Part print with two shaded views. Sizes in mm from the minimum x, y, z corner. A direction names the side the tool comes from. Round coordinates to 2 decimals unless told otherwise and drop trailing zeros. Order: outer loops, then holes, each group sorted by start corner. A loop starts at its lowest first (then second) coordinate and runs counter-clockwise, first axis right, second up. Notation, with made-up numbers: M 12.25,84 L 21.25,84 A10 cw 21.25,102 Z; hole C 4.25,88 d4. An arc over 180 degrees is marked long. Put each result on its own line as item: value.
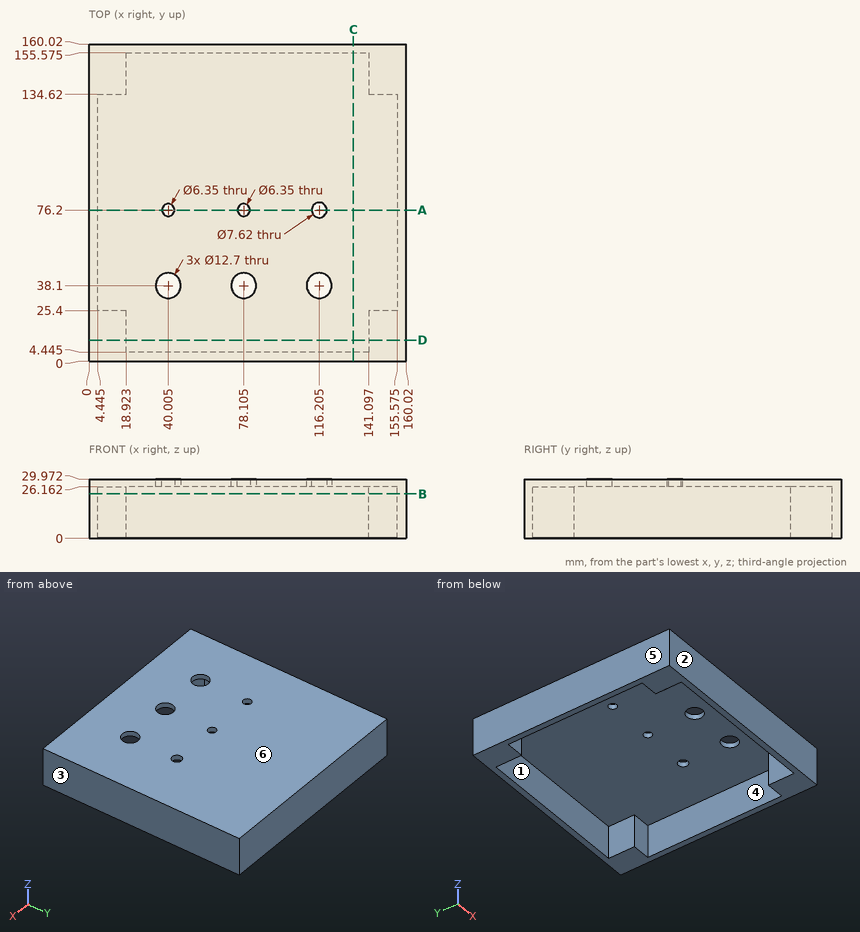
Item 1: Band-saw the part on D-D on y = 10.5. Give the cut face in (x, z), and give its area (3 significant figures).
Answers below:
outline: M 0,0 L 18.92,0 L 18.92,26.16 L 141.1,26.16 L 141.1,0 L 160.02,0 L 160.02,29.97 L 0,29.97 Z
area: 1,600 mm²
Item 2: Band-saw the part on A-A on y = 76.2. Give the cut face in (x, z) (3 decimals).
Answers below:
outline: M 0,0 L 4.445,0 L 4.445,26.162 L 36.83,26.162 L 36.83,29.972 L 0,29.972 Z; M 43.18,26.162 L 74.93,26.162 L 74.93,29.972 L 43.18,29.972 Z; M 81.28,26.162 L 112.395,26.162 L 112.395,29.972 L 81.28,29.972 Z; M 120.015,26.162 L 155.575,26.162 L 155.575,0 L 160.02,0 L 160.02,29.972 L 120.015,29.972 Z
Item 3: Tool access for the marked faces 1 and 2: list every direction of +Z, -Z, +X, -X, +Y, -Y with a clear straight run to the whole face (end or side of a thin tool).
Answers below:
face 1: -Z
face 2: +Z, -Z, +X, -X, -Y
Item 4: Probe line 1 along Y through (x, z) = (150, 14.5); line 2 along Y through (x, z) = (73.5, 2.5) (3 decimals). List the from-to ranges inside material, lowest first. Write a range as [from, to].
Answers below:
line 1: [0, 25.4], [134.62, 160.02]
line 2: [0, 4.445], [155.575, 160.02]
Item 5: Pin check, flat tips, straight feed: P1, Ø8, axis at x = 76.5, y = 35, coming from the +Z side; P2, Ø8, axis at x = 119, y = 142.5, coming from the -Z side; P3, Ø7.5, axis at x = 116.205, y = 38.1, coming from the -Z side. Stop position of each tip, or through.
Answers below:
P1: z = 29.97
P2: z = 26.16
P3: through
Item 6: Mould opens along X. For the marked faces 3, 4, 5 and 6 say: pulls with the +X half, pulls with the -X half, needs draft (parallel to the pull), parting line crosses it, or undercut.
Answers below:
face 3: pulls with the +X half
face 4: undercut
face 5: pulls with the -X half
face 6: needs draft
Item 7: Band-saw the part on C-C on x = 133.5. Give the cut face in (y, z) (3 decimals).
Answers below:
outline: M 0,0 L 4.445,0 L 4.445,26.162 L 155.575,26.162 L 155.575,0 L 160.02,0 L 160.02,29.972 L 0,29.972 Z
Item 8: Band-saw the part on B-B on z = 22.5. Give the cut face in (x, y) (3 decimals).
Answers below:
outline: M 0,0 L 160.02,0 L 160.02,160.02 L 0,160.02 Z; hole M 4.445,25.4 L 18.923,25.4 L 18.923,4.445 L 141.097,4.445 L 141.097,25.4 L 155.575,25.4 L 155.575,134.62 L 141.097,134.62 L 141.097,155.575 L 18.923,155.575 L 18.923,134.62 L 4.445,134.62 Z
